The model under review builds one solid part; all positions refer to its coordinate system, in mm. Coordinates: 2 decimals unless noted, no trailing zeros. Loops run counter-clockwise (first coordinate to the right, second up) from the corner with the lowest first, then second, coordinate; pieces in that order, holes last. Notation, with made-up numbers: (62, -13) - (100, -13) arc R22 cw to (100, 11) - close; hole circle Ø1 at (-28.75, 58.5). An arc over 180 degrees is marked (long way). Use a Markdown table: item, result. Add a question column.
1) Add section D-D, the plane x = 5. Give the boundary of the cut face in (y, z).
2) Clearance check with flat-ended pins moving along their axes: pin 1 (11.5 mm diameter, centred on x = 12.5, z = -14, fed in from +Y); pin 2 (0.5 mm diameter, centred on y = 3, z = -12, fed in from -X); pin 3 (1.5 mm diameter, centred on y = 2, z = -20.5, fed in from +X); pin 4 (0.5 mm diameter, centred on y = 2, z = -11, fed in from +X). State where each tip first meets the part, or that it passes through.
3) Add section B-B, the plane y = 0.7. Give the boundary of the cut face in (x, z).
4) To check wall thickness, follow L1, parallel to X at y = 0.9, z = -19.7; L2, parallel to Z at x = 18.25, y = 0.5; L3, parallel to Y at x = 17.5, z = -12.25. State the ranges of each line that lie inside material, in increasing order. Write a range as [from, to].
5) Add section C-C, the plane z = -11.7. Give the boundary of the cut face in (x, y), and give its area (3 significant figures).
6) Add section A-A, the plane x = 11.7. Give the boundary of the cut face in (y, z).
```python
from build123d import *

# Parameters (mm, degrees)
SKETCH1_R           = 1.75
BOSS_EXTRUDE1_DEPTH = 1.6
SKETCH2_W           = 2
SKETCH2_H           = 5
BOSS_EXTRUDE2_DEPTH = 1.7
SKETCH3_R           = 1.5
BOSS_EXTRUDE3_DEPTH = 0.3


with BuildPart() as part:
    # Sketch1 → Boss-Extrude1 (new body)
    with BuildSketch(Plane(origin=(0, 0, 0), x_dir=(1, 0, 0), z_dir=(0, 1, 0))):
        with BuildLine():
            Line((3.7, 0), (19.7, 0))
            ThreePointArc((19.7, 0), (22.31629509, 1.08370491), (23.4, 3.7))
            Line((23.4, 3.7), (23.4, 19.7))
            ThreePointArc((23.4, 19.7), (22.31629509, 22.31629509), (19.7, 23.4))
            Line((19.7, 23.4), (3.7, 23.4))
            ThreePointArc((3.7, 23.4), (1.08370491, 22.31629509), (0, 19.7))
            Line((0, 19.7), (0, 3.7))
            ThreePointArc((0, 3.7), (1.08370491, 1.08370491), (3.7, 0))
        make_face()
        with Locations(Location((3.7, 19.7, 0), (0, 0, 270))):
            Circle(SKETCH1_R, mode=Mode.SUBTRACT)
        with Locations(Location((19.7, 19.7, 0), (0, 0, 270))):
            Circle(SKETCH1_R, mode=Mode.SUBTRACT)
        with Locations(Location((19.7, 3.7, 0), (0, 0, 270))):
            Circle(SKETCH1_R, mode=Mode.SUBTRACT)
        with Locations(Location((3.7, 3.7, 0), (0, 0, 270))):
            Circle(SKETCH1_R, mode=Mode.SUBTRACT)
    extrude(amount=BOSS_EXTRUDE1_DEPTH)

    # Sketch2 → Boss-Extrude2 (add)
    with BuildSketch(Plane(origin=(0, 1.6, 0), x_dir=(1, 0, 0), z_dir=(0, 1, 0))):
        with Locations((12.7, 11.7)):
            Rectangle(SKETCH2_W, SKETCH2_H)
        with Locations((10.7, 11.7)):
            Rectangle(SKETCH2_W, SKETCH2_H)
    extrude(amount=BOSS_EXTRUDE2_DEPTH)

    # Sketch3 → Boss-Extrude3 (add)
    with BuildSketch(Plane(origin=(0, 3.3, 0), x_dir=(1, 0, 0), z_dir=(0, 1, 0))):
        with Locations(Location((11.7, 11.7, 0), (0, 0, 270))):
            Circle(SKETCH3_R)
    extrude(amount=BOSS_EXTRUDE3_DEPTH)


solid = part.part
```
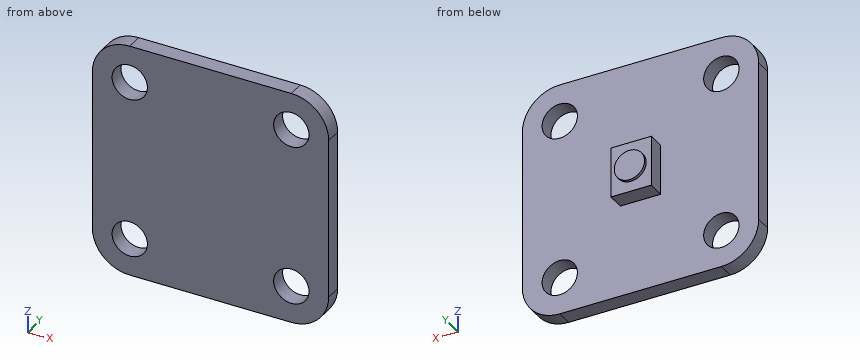
From the geometry:
| question | item | result |
|---|---|---|
| 1 | outline | (0, -23.4) - (1.6, -23.4) - (1.6, -20.87) - (0, -20.87) - close; (0, -18.53) - (1.6, -18.53) - (1.6, -4.87) - (0, -4.87) - close; (0, -2.53) - (1.6, -2.53) - (1.6, 0) - (0, 0) - close |
| 2 | pin 1 | stops at y = 3.6 |
| 2 | pin 2 | stops at x = 9.7 |
| 2 | pin 3 | stops at x = 23.4 |
| 2 | pin 4 | stops at x = 13.7 |
| 3 | outline | (0, -19.7) arc R3.7 ccw to (3.7, -23.4) - (19.7, -23.4) arc R3.7 ccw to (23.4, -19.7) - (23.4, -3.7) arc R3.7 ccw to (19.7, 0) - (3.7, 0) arc R3.7 ccw to (0, -3.7) - close; hole circle Ø3.5 at (3.7, -19.7); hole circle Ø3.5 at (3.7, -3.7); hole circle Ø3.5 at (19.7, -19.7); hole circle Ø3.5 at (19.7, -3.7) |
| 4 | L1 | x = [0, 1.95], [5.45, 17.95], [21.45, 23.4] |
| 4 | L2 | z = [-23.4, -20.68], [-18.72, -4.68], [-2.72, 0] |
| 4 | L3 | y = [0, 1.6] |
| 5 | outline | (0, 0) - (23.4, 0) - (23.4, 1.6) - (13.7, 1.6) - (13.7, 3.3) - (13.2, 3.3) - (13.2, 3.6) - (10.2, 3.6) - (10.2, 3.3) - (9.7, 3.3) - (9.7, 1.6) - (0, 1.6) - close |
| 5 | area | 45.1 mm^2 |
| 6 | outline | (0, -23.4) - (1.6, -23.4) - (1.6, -14.2) - (3.3, -14.2) - (3.3, -13.2) - (3.6, -13.2) - (3.6, -10.2) - (3.3, -10.2) - (3.3, -9.2) - (1.6, -9.2) - (1.6, 0) - (0, 0) - close |
